Can you work these out from the model? Positions are in its coordinate system, mm. A direction names the side the tool comes from. Give positions to 0.01 mm unless a question says otherwise; leave off trailing zeros. Order: outer loops, then holes, each group sorted by start corner. A loop starts at its lowest first (then second) coordinate and runs counter-clockwise, first axis right, second up. Notation, with made-up numbers: M -35.5,-5.5 L 6.5,-5.5 A14 cw 6.5,19.5 Z; hole C 12,76.25 d4. An arc over 180 degrees is marked long. One line per question, with ' | ' between items. Start each with the question number.
1) Please list where these lines run through material, in increasing order: line 1 along Y through (x, z) = (7.5, 12.3); line 2 along Z through (x, y) = (30.5, 3.5); line 3 along Y through (x, z) = (48, 5.75). Write a range as [from, to].
2) For faces 1 (the cylindrical face through (8.65, 5.28, 11.48)), 2 (the flat face through (25, 0, 5)), which set-ups out of +Z, -Z, +X, -X, +Y, -Y let a thin tool reach every point of the face, with its end or its side?
3) I'm going to push flat-ended pins straight in: pin 1 Ø1.5 at (x, y) = (8.5, 7) entering from +Z; pin 2 Ø6 at (y, z) = (2, 5) entering from +X; pin 3 Ø6 at (x, y) = (7.5, 7.5) entering from -Z. Where does each tip first touch, or does it pass through?
4) If we section it at C-C, the plane z = 11.75: Please give me the cut outline in (x, y).
5) Thinking about a two-plate mould opening in X: for faces 3 (the cylindrical face through (10.997, 7.346, 11.479)), 4 (the flat face through (7, 8, 10)), 5 (the flat face through (25, 8, 10)), which applies, +X half, -X half, draft (parallel to the pull), parting line (faces both ways), or undercut?
6) If we section it at B-B, the plane x = 35.5: Please give me the cut outline in (y, z).
7) If we section it at D-D, the plane y = 1: Please give me the cut outline in (x, z).
```python
from build123d import *

# Parameters (mm, degrees)
SKETCH1_W           = 50
SKETCH1_H           = 15
BOSS_EXTRUDE1_DEPTH = 10
FILLET1_R           = 7.5
SKETCH2_R           = 3.5
SKETCH2_R_2         = 2.5
BOSS_EXTRUDE2_DEPTH = 3


with BuildPart() as part:
    # Sketch1 → Boss-Extrude1 (new body)
    with BuildSketch(Plane.XY):
        with Locations((25, 7.5)):
            Rectangle(SKETCH1_W, SKETCH1_H)
    extrude(amount=BOSS_EXTRUDE1_DEPTH)

    # Fillet1
    fillet1_edges = [part.edges().sort_by_distance(p)[0] for p in [
        (50, 0, 5),
        (50, 15, 5),
        (0, 0, 5),
        (0, 15, 5),
    ]]
    fillet(fillet1_edges, radius=FILLET1_R - 0.0001)  # a hair under: the kernel refuses the full size

    # Sketch2 → Boss-Extrude2 (add)
    with BuildSketch(Plane.XY.offset(10)):
        with Locations(Location((7.5, 7.5, 0), (0, 0, 180))):
            Circle(SKETCH2_R)
        with Locations((7.5, 7.5)):
            Circle(SKETCH2_R_2, mode=Mode.SUBTRACT)
    extrude(amount=BOSS_EXTRUDE2_DEPTH)


solid = part.part
```
Results found:
1) line 1: y = [4, 5], [10, 11] | line 2: z = [0, 10] | line 3: y = [2.4, 12.6]
2) face 1: +Z | face 2: +Z, -Z, +X, -X, -Y
3) pin 1: stops at z = 10 | pin 2: stops at x = 49.57 | pin 3: stops at z = 0
4) outline: C 7.5,7.5 d7; hole C 7.5,7.5 d5
5) face 3: parting line | face 4: undercut | face 5: draft
6) outline: M 0,0 L 15,0 L 15,10 L 0,10 Z
7) outline: M 3.76,0 L 46.24,0 L 46.24,10 L 3.76,10 Z
